Geometry: final body of the model. Coordinates: model frame, mm. A direction names the side the tool comes from. Coordinates: 2 decimals unless noted, no trailing zeros. Order: outer loops, then holes, each group sorted by start corner. A loop starts at its lowest first (then second) coordinate and runs counter-clockwise, first axis right, second up. Notation, with made-up numbers: M 57.5,42.25 L 81.5,42.25 A20 cw 81.5,46.25 Z; hole C 73,-27 d8. An arc over 180 degrees is marked long. Use CSV: the item, a comma, the result in double quotes. Start each with the question number.
Q1. Access query for faces 5 (the face through (62, 95, 58)), 6 (the face through (-30, 54, 49)), 7 (the face through (21, 11.694, 58)). Directions: +Z, -Z, +X, -X, +Y, -Y. A direction counts if a zero-diameter tool reaches every point of the face in a straight line with its end or side. Return the directions, or none.
Q2. Section query D-D, the plane y = 29.5. Output: boundary loops of the cut face in (x, z), and give its area (3 significant figures).
Q3. Mould query, pull axis X, two halves, no side actions, for faces 1 (the face through (-75, 49, 53)), 2 (the face through (75, 49, 58)), 3 (the face through (-35, 89, 57)), 4 (the face through (30, 55.5, 49)). Classes: +X half, -X half, draft (parallel to the pull), parting line (faces both ways), or undercut.
Q4. Section query B-B, the plane y = 41.75. Output: boundary loops of the cut face in (x, z), and give its area (3 significant figures).
Q5. Ray query, probe 1 along Y at (x, z) = (-65, 59.5); probe 2 along Y at (x, z) = (60, 56.75); probe 3 along X at (y, z) = (95, 56.5). Return the intervals inside material, ascending.
Q6. Section query C-C, the plane x = -65. Output: boundary loops of the cut face in (y, z), and give its area (3 significant figures).
Q7. First-contact query: P1, Ø7.5, axis at x = 26, z = 45, coming from the -Y side; P2, Ø7.5, axis at x = 56, y = 5, coming from the +Z side; P3, Ø3, axis at x = 15.5, y = 39.5, coming from the -Z side; P4, Ø1.6, axis at y = 54.5, z = 51.5, coming from the +X side. Flat tips, straight axial feed; report the tip coordinate or a pass-through.
Q8. Section query A-A, the plane x = -15. Output: boundary loops of the cut face in (y, z).
from build123d import *

# Parameters (mm, degrees)
SKETCH1_W                 = 150
SKETCH1_H                 = 4
BOSS_EXTRUDE1_DEPTH       = 100
CUT_EXTRUDE1_REACH        = 127.064
SKETCH7_W                 = 57
SKETCH7_H                 = 11.694235649
SKETCH9_W                 = 4
SKETCH9_H                 = 100
BOSS_EXTRUDE4_DEPTH       = 11
SKETCH10_W                = 20
SKETCH10_H                = 1.5
BOSS_EXTRUDE5_DEPTH       = 15
LPATTERN1_COUNT           = 2
LPATTERN1_PITCH           = 60
LPATTERN2_COUNT           = 2
LPATTERN2_PITCH           = 25
LPATTERN2_COPY_1_SKETCH_W = 20
LPATTERN2_COPY_1_SKETCH_H = 1.5
LPATTERN2_COPY_1_DEPTH    = 15
LPATTERN3_COUNT           = 2
LPATTERN3_PITCH           = 4
LPATTERN3_COPY_1_SKETCH_W = 20
LPATTERN3_COPY_1_SKETCH_H = 1.5
LPATTERN3_COPY_1_DEPTH    = 15
LPATTERN3_COPY_2_SKETCH_W = 20
LPATTERN3_COPY_2_SKETCH_H = 1.5
LPATTERN3_COPY_2_DEPTH    = 15
LPATTERN3_COPY_3_SKETCH_W = 20
LPATTERN3_COPY_3_SKETCH_H = 1.5
LPATTERN3_COPY_3_DEPTH    = 15
SKETCH12_R                = 3.5
CUT_EXTRUDE2_DEPTH        = 2
CUT_EXTRUDE3_REACH        = 128.151
SKETCH13_R                = 2.25
LPATTERN4_COUNT           = 2
LPATTERN4_PITCH           = 50
SKETCH15_R                = 3
CUT_EXTRUDE4_DEPTH        = 2
CUT_EXTRUDE5_REACH        = 219.319
SKETCH17_R                = 1.75
LPATTERN5_COUNT           = 2
LPATTERN5_PITCH           = 25
SKETCH18_W                = 10
SKETCH18_H                = 7
CUT_EXTRUDE6_DEPTH        = 3
LPATTERN6_COUNT           = 2
LPATTERN6_PITCH           = 55
CUT_EXTRUDE7_REACH        = 127.897
SKETCH19_W                = 11
SKETCH19_H                = 68.305764351
FILLET1_R                 = 2
LPATTERN7_COUNT           = 3
LPATTERN7_PITCH           = 50
FILLET1_OF_LPATTERN7_R    = 2
LPATTERN8_COUNT           = 2
LPATTERN8_PITCH           = 120
SKETCH20_W                = 8
SKETCH20_H                = 10
CUT_EXTRUDE8_DEPTH        = 3
LPATTERN9_COUNT           = 2
LPATTERN9_PITCH           = 60
SKETCH22_R                = 3
CUT_EXTRUDE9_DEPTH        = 2
CUT_EXTRUDE10_REACH       = 217.691
SKETCH24_R                = 1.75
SKETCH26_R                = 3
CUT_EXTRUDE11_DEPTH       = 2
CUT_EXTRUDE12_REACH       = 123.185
SKETCH28_R                = 1.75
LPATTERN11_COUNT          = 2
LPATTERN11_PITCH          = 125


with BuildPart() as part:
    # Sketch1 → Boss-Extrude1 (new body)
    with BuildSketch(Plane(origin=(0, 0, 0), x_dir=(1, 0, 0), z_dir=(0, 1, 0))):
        with Locations((0, -58)):
            Rectangle(SKETCH1_W, SKETCH1_H)
    extrude(amount=BOSS_EXTRUDE1_DEPTH)

    # Sketch7 → Cut-Extrude1 (cut, up to next)
    with BuildSketch(Plane.XY.offset(60), mode=Mode.PRIVATE) as cut_extrude1_sk1:
        with Locations((21.68, 5.847117825)):
            Rectangle(SKETCH7_W, SKETCH7_H)
    cut_extrude1_tool1 = extrude(cut_extrude1_sk1.sketch, amount=-CUT_EXTRUDE1_REACH, mode=Mode.PRIVATE) & part.part
    add(cut_extrude1_tool1.solids().sort_by_distance((21.68, 5.847118, 60))[0], mode=Mode.SUBTRACT)

    # Sketch9 → Boss-Extrude4 (add)
    with BuildSketch(Plane(origin=(0, 0, 56), x_dir=(-1, 0, 0), z_dir=(0, 0, -1))):
        with Locations((73, 50)):
            Rectangle(SKETCH9_W, SKETCH9_H)
    extrude(amount=BOSS_EXTRUDE4_DEPTH)

    # Sketch10 → Boss-Extrude5 (add)
    with BuildSketch(Plane(origin=(0, 0, 56), x_dir=(-1, 0, 0), z_dir=(0, 0, -1))):
        with Locations((-30, 50.75)):
            Rectangle(SKETCH10_W, SKETCH10_H)
    boss_extrude5 = extrude(amount=BOSS_EXTRUDE5_DEPTH)

    # LPattern1: Boss-Extrude5 ×2
    with Locations(*[(-i * LPATTERN1_PITCH, 0, 0) for i in range(1, LPATTERN1_COUNT)]):
        add(boss_extrude5)

    # LPattern2: Boss-Extrude5 ×2
    with Locations(*[(0, i * LPATTERN2_PITCH, 0) for i in range(1, LPATTERN2_COUNT)]):
        add(boss_extrude5)

    # LPattern2 copy 1 sketch → LPattern2 copy 1 (add)
    with BuildSketch(Plane(origin=(-60, 25, 56), x_dir=(-1, 0, 0), z_dir=(0, 0, -1))):
        with Locations((-30, 50.75)):
            Rectangle(LPATTERN2_COPY_1_SKETCH_W, LPATTERN2_COPY_1_SKETCH_H)
    extrude(amount=LPATTERN2_COPY_1_DEPTH)

    # LPattern3: Boss-Extrude5 ×2
    with Locations(*[(0, i * LPATTERN3_PITCH, 0) for i in range(1, LPATTERN3_COUNT)]):
        add(boss_extrude5)

    # LPattern3 copy 1 sketch → LPattern3 copy 1 (add)
    with BuildSketch(Plane(origin=(-60, 4, 56), x_dir=(-1, 0, 0), z_dir=(0, 0, -1))):
        with Locations((-30, 50.75)):
            Rectangle(LPATTERN3_COPY_1_SKETCH_W, LPATTERN3_COPY_1_SKETCH_H)
    extrude(amount=LPATTERN3_COPY_1_DEPTH)

    # LPattern3 copy 2 sketch → LPattern3 copy 2 (add)
    with BuildSketch(Plane(origin=(0, 29, 56), x_dir=(-1, 0, 0), z_dir=(0, 0, -1))):
        with Locations((-30, 50.75)):
            Rectangle(LPATTERN3_COPY_2_SKETCH_W, LPATTERN3_COPY_2_SKETCH_H)
    extrude(amount=LPATTERN3_COPY_2_DEPTH)

    # LPattern3 copy 3 sketch → LPattern3 copy 3 (add)
    with BuildSketch(Plane(origin=(-60, 29, 56), x_dir=(-1, 0, 0), z_dir=(0, 0, -1))):
        with Locations((-30, 50.75)):
            Rectangle(LPATTERN3_COPY_3_SKETCH_W, LPATTERN3_COPY_3_SKETCH_H)
    extrude(amount=LPATTERN3_COPY_3_DEPTH)

    # Sketch12 → Cut-Extrude2 (cut)
    with BuildSketch(Plane.XY.offset(60)):
        with Locations((-65, 6)):
            Circle(SKETCH12_R)
    cut_extrude2 = extrude(amount=-CUT_EXTRUDE2_DEPTH, mode=Mode.SUBTRACT)

    # Sketch13 → Cut-Extrude3 (cut, up to next)
    with BuildSketch(Plane.XY.offset(58), mode=Mode.PRIVATE) as cut_extrude3_sk1:
        with Locations((-65, 6)):
            Circle(SKETCH13_R)
    cut_extrude3_tool1 = extrude(cut_extrude3_sk1.sketch, amount=-CUT_EXTRUDE3_REACH, mode=Mode.PRIVATE) & part.part
    cut_extrude3 = cut_extrude3_tool1.solids().sort_by_distance((-65, 6, 58))[0]
    add(cut_extrude3, mode=Mode.SUBTRACT)

    # LPattern4: Cut-Extrude2, Cut-Extrude3 ×2
    with Locations(*[(i * LPATTERN4_PITCH, 0, 0) for i in range(1, LPATTERN4_COUNT)]):
        add(cut_extrude2, mode=Mode.SUBTRACT)
        add(cut_extrude3, mode=Mode.SUBTRACT)

    # Sketch15 → Cut-Extrude4 (cut)
    with BuildSketch(Plane(origin=(125.77806455, 81.403570161, 60), x_dir=(1, 0, 0), z_dir=(0, 0, 1))):
        with Locations((-65.77806455, 0.346429839)):
            Circle(SKETCH15_R)
    cut_extrude4 = extrude(amount=-CUT_EXTRUDE4_DEPTH, mode=Mode.SUBTRACT)

    # Sketch17 → Cut-Extrude5 (cut, up to next)
    with BuildSketch(Plane(origin=(125.77806455, 81.403570161, 58), x_dir=(1, 0, 0), z_dir=(0, 0, 1)), mode=Mode.PRIVATE) as cut_extrude5_sk1:
        with Locations((-65.77806455, 0.346429839)):
            Circle(SKETCH17_R)
    cut_extrude5_tool1 = extrude(cut_extrude5_sk1.sketch, amount=-CUT_EXTRUDE5_REACH, mode=Mode.PRIVATE) & part.part
    cut_extrude5 = cut_extrude5_tool1.solids().sort_by_distance((60, 81.75, 58))[0]
    add(cut_extrude5, mode=Mode.SUBTRACT)

    # LPattern5: Cut-Extrude4, Cut-Extrude5 ×2
    with Locations(*[(0, -i * LPATTERN5_PITCH, 0) for i in range(1, LPATTERN5_COUNT)]):
        add(cut_extrude4, mode=Mode.SUBTRACT)
        add(cut_extrude5, mode=Mode.SUBTRACT)

    # Sketch18 → Cut-Extrude6 (cut)
    with BuildSketch(Plane(origin=(0, 0, 56), x_dir=(-1, 0, 0), z_dir=(0, 0, -1))):
        with Locations((-67.5, 86.5)):
            Rectangle(SKETCH18_W, SKETCH18_H)
    cut_extrude6 = extrude(amount=-CUT_EXTRUDE6_DEPTH, mode=Mode.SUBTRACT)

    # LPattern6: Cut-Extrude6 ×2
    with Locations(*[(0, -i * LPATTERN6_PITCH, 0) for i in range(1, LPATTERN6_COUNT)]):
        add(cut_extrude6, mode=Mode.SUBTRACT)

    # Sketch19 → Cut-Extrude7 (cut, up to next)
    with BuildSketch(Plane(origin=(0, 0, 56), x_dir=(-1, 0, 0), z_dir=(0, 0, -1)), mode=Mode.PRIVATE) as cut_extrude7_sk1:
        with Locations((-49, 55.847117825)):
            Rectangle(SKETCH19_W, SKETCH19_H)
    cut_extrude7_tool1 = extrude(cut_extrude7_sk1.sketch, amount=-CUT_EXTRUDE7_REACH, mode=Mode.PRIVATE) & part.part
    cut_extrude7 = cut_extrude7_tool1.solids().sort_by_distance((49, 55.847118, 56))[0]
    add(cut_extrude7, mode=Mode.SUBTRACT)

    # Fillet1
    fillet1_edges = [part.edges().sort_by_distance(p)[0] for p in [
        (54.5, 21.694235649, 58),
        (54.5, 90, 58),
        (43.5, 90, 58),
        (43.5, 21.694235649, 58),
    ]]
    fillet(fillet1_edges, radius=FILLET1_R)

    # LPattern7: Cut-Extrude7 ×3
    with Locations(*[(-i * LPATTERN7_PITCH, 0, 0) for i in range(1, LPATTERN7_COUNT)]):
        add(cut_extrude7, mode=Mode.SUBTRACT)

    # Fillet1 of LPattern7
    fillet1_of_lpattern7_edges = [part.edges().sort_by_distance(p)[0] for p in [
        (4.5, 21.694235649, 58),
        (4.5, 90, 58),
        (-6.5, 90, 58),
        (-6.5, 21.694235649, 58),
        (-45.5, 21.694235649, 58),
        (-45.5, 90, 58),
        (-56.5, 90, 58),
        (-56.5, 21.694235649, 58),
    ]]
    fillet(fillet1_of_lpattern7_edges, radius=FILLET1_OF_LPATTERN7_R)

    # LPattern8: Cut-Extrude2, Cut-Extrude3 ×2
    with Locations(*[(i * LPATTERN8_PITCH, 0, 0) for i in range(1, LPATTERN8_COUNT)]):
        add(cut_extrude2, mode=Mode.SUBTRACT)
        add(cut_extrude3, mode=Mode.SUBTRACT)

    # Sketch20 → Cut-Extrude8 (cut)
    with BuildSketch(Plane(origin=(0, 0, 56), x_dir=(-1, 0, 0), z_dir=(0, 0, -1))):
        with Locations((-29, 89.134967696)):
            Rectangle(SKETCH20_W, SKETCH20_H)
    cut_extrude8 = extrude(amount=-CUT_EXTRUDE8_DEPTH, mode=Mode.SUBTRACT)

    # LPattern9: Cut-Extrude8 ×2
    with Locations(*[(-i * LPATTERN9_PITCH, 0, 0) for i in range(1, LPATTERN9_COUNT)]):
        add(cut_extrude8, mode=Mode.SUBTRACT)

    # Sketch22 → Cut-Extrude9 (cut)
    with BuildSketch(Plane(origin=(131.167270466, 38.938204498, 60), x_dir=(1, 0, 0), z_dir=(0, 0, 1))):
        with Locations((-62.167270466, 2.811795502)):
            Circle(SKETCH22_R)
    extrude(amount=-CUT_EXTRUDE9_DEPTH, mode=Mode.SUBTRACT)

    # Sketch24 → Cut-Extrude10 (cut, up to next)
    with BuildSketch(Plane(origin=(131.167270466, 38.938204498, 58), x_dir=(1, 0, 0), z_dir=(0, 0, 1)), mode=Mode.PRIVATE) as cut_extrude10_sk1:
        with Locations((-62.167270466, 2.811795502)):
            Circle(SKETCH24_R)
    cut_extrude10_tool1 = extrude(cut_extrude10_sk1.sketch, amount=-CUT_EXTRUDE10_REACH, mode=Mode.PRIVATE) & part.part
    add(cut_extrude10_tool1.solids().sort_by_distance((69, 41.75, 58))[0], mode=Mode.SUBTRACT)

    # Sketch26 → Cut-Extrude11 (cut)
    with BuildSketch(Plane(origin=(-1.555186457, 92.391705768, 60), x_dir=(1, 0, 0), z_dir=(0, 0, 1))):
        with Locations((-63.444813543, 2.608294232)):
            Circle(SKETCH26_R)
    cut_extrude11 = extrude(amount=-CUT_EXTRUDE11_DEPTH, mode=Mode.SUBTRACT)

    # Sketch28 → Cut-Extrude12 (cut, up to next)
    with BuildSketch(Plane(origin=(-1.555186457, 92.391705768, 58), x_dir=(1, 0, 0), z_dir=(0, 0, 1)), mode=Mode.PRIVATE) as cut_extrude12_sk1:
        with Locations((-63.444813543, 2.608294232)):
            Circle(SKETCH28_R)
    cut_extrude12_tool1 = extrude(cut_extrude12_sk1.sketch, amount=-CUT_EXTRUDE12_REACH, mode=Mode.PRIVATE) & part.part
    cut_extrude12 = cut_extrude12_tool1.solids().sort_by_distance((-65, 95, 58))[0]
    add(cut_extrude12, mode=Mode.SUBTRACT)

    # LPattern11: Cut-Extrude11, Cut-Extrude12 ×2
    with Locations(*[(i * LPATTERN11_PITCH, 0, 0) for i in range(1, LPATTERN11_COUNT)]):
        add(cut_extrude11, mode=Mode.SUBTRACT)
        add(cut_extrude12, mode=Mode.SUBTRACT)


solid = part.part
Responses:
1,face 5,"+Z"
1,face 6,"-Z, +X"
1,face 7,"+Z, -Z, -Y"
2,outline,"M -75,45 L -71,45 L -71,56 L -56.5,56 L -56.5,60 L -75,60 Z; M -45.5,56 L -6.5,56 L -6.5,60 L -45.5,60 Z; M 4.5,56 L 43.5,56 L 43.5,60 L 4.5,60 Z; M 54.5,56 L 62.5,56 L 62.5,59 L 72.5,59 L 72.5,56 L 75,56 L 75,60 L 54.5,60 Z"
2,area,"482 mm²"
3,face 1,"-X half"
3,face 2,"+X half"
3,face 3,"undercut"
3,face 4,"draft"
4,outline,"M -75,45 L -71,45 L -71,56 L -56.5,56 L -56.5,60 L -75,60 Z; M -45.5,56 L -6.5,56 L -6.5,60 L -45.5,60 Z; M 4.5,56 L 43.5,56 L 43.5,60 L 4.5,60 Z; M 54.5,56 L 67.25,56 L 67.25,58 L 66,58 L 66,60 L 54.5,60 Z; M 70.75,56 L 75,56 L 75,60 L 72,60 L 72,58 L 70.75,58 Z"
4,area,"493 mm²"
5,probe 1,"y = 0 to 2.5, 9.5 to 92, 98 to 100"
5,probe 2,"y = 0 to 55, 58.5 to 80, 83.5 to 93.25, 96.75 to 100"
5,probe 3,"x = -75 to -66.75, -63.25 to 58.25, 61.75 to 75"
6,outline,"M 0,56 L 3.75,56 L 3.75,58 L 2.5,58 L 2.5,60 L 0,60 Z; M 8.25,56 L 93.25,56 L 93.25,58 L 92,58 L 92,60 L 9.5,60 L 9.5,58 L 8.25,58 Z; M 96.75,56 L 100,56 L 100,60 L 98,60 L 98,58 L 96.75,58 Z"
6,area,"358 mm²"
7,P1,"stops at y = 50"
7,P2,"stops at z = 60"
7,P3,"stops at z = 56"
7,P4,"stops at x = 40"
8,outline,"M 0,56 L 3.75,56 L 3.75,58 L 2.5,58 L 2.5,60 L 0,60 Z; M 8.25,56 L 100,56 L 100,60 L 9.5,60 L 9.5,58 L 8.25,58 Z"
